```python
from build123d import *

# Parameters (mm, degrees)
F1_DEPTH      = 25.4
F2_T          = -2.54
F8_DEPTH      = 12.7
F8_DEPTH_BACK = 25.4


# Not quite as in the source:
# - the program builds the solid bodies; features that only make, move or delete a surface that nothing else refers to are left out


with BuildPart() as f1:
    # F0 (on Top) → F1 (new body)
    with BuildSketch(Plane.XY):
        Polygon((10.2551429075, 58.9377772835), (-40.5448570925, 58.9377772835), (-71.7704754875, 18.8678289949), (-41.2404706852, -21.7346192906), (9.5595293148, -21.7346192906), (40.7851477097, 18.335328998), align=None)
    extrude(amount=F1_DEPTH)

    # F2
    f2_openings = [f1.faces().sort_by_distance(p)[0] for p in [
        (-15.492664, 18.601579, 25.4),
    ]]
    offset(amount=F2_T, openings=f2_openings)

    # F7 (on Top) → F8 (join, two sides)
    with BuildSketch(Plane.XY) as f8_sk:
        Polygon((0, 0), (-50.8, 0), (-38.1, -21.9970452561), (-12.7, -21.9970452561), align=None)
    extrude(amount=F8_DEPTH)
    extrude(f8_sk.sketch, amount=-F8_DEPTH_BACK)


solid = f1.part
```
Build history of the part. All positions in model axes, mm. A direction names the side the tool comes from. Give positions to 0.01 mm unless a question says otherwise; leave off trailing zeros. Order: outer loops, then holes, each group sorted by start corner. A loop starts at its lowest first (then second) coordinate and runs counter-clockwise, first axis right, second up. Notation, with made-up numbers: M 30,89.25 L 61,89.25 A29 ccw 61,117.25 Z; hole C -20.5,41 d11. An arc over 180 degrees is marked long. Write item = value, one per line. Start each with the question number.
(1) Slice it at D-D on z = -14.5. Write the cut outline in (x, y).
(2) Probe L1, parallel to Z at x = -57.5, y = 33.5; L2, parallel to Z at x = 20, y = 23.5; L3, parallel to Y at x = -36, z = -14. List the from-to ranges inside material, lowest first. Write a range as [from, to].
(3) Pin check, flat tips, straight feed: pin 1 Ø1.5 at (y, z) = (30, 13.5) entering from -X; pin 2 Ø2 at (y, z) = (-11, -0.5) entering from -X; pin 3 Ø4 at (x, z) = (-39, -14.5) entering from +Y. Stop position of each tip, or through.
(4) Which spindle directions (+Z, -Z, +X, -X, +Y, -Y) get a long thin tool onto all of the face, cutting with end or side? Do faces 1 (the flat face through (-54.472, 0.089, 13.81)), 2 (the flat face through (-15, 58.938, 13)), 3 (the flat face through (-25, 0, -13)). Say none if no direction does.
(5) Slice it at A-A on z = 7. Write the cut outline in (x, y), plus the area to 3 significant figures.
(6) Slice it at B-B on x = -36. Write the cut outline in (y, z).
(7) Two-plate mould, pull along X, no slides. Class faces 4 (the flat face through (-16, 58, 25.4)), 5 (the flat face through (-55.94, 39.18, 12.52)), 6 (the flat face through (22.748, -0.679, 13.81)): released by +X, released by -X, zero draft, split by the parting line, or undercut.
(8) Slice it at C-C on y = 28.5. Write the cut outline in (x, z), plus the area to 3 significant figures.
Responses:
q1.outline = M -50.8,0 L -38.1,-22 L -12.7,-22 L 0,0 Z
q2.L1 = [0, 25.4]
q2.L2 = [0, 2.54]
q2.L3 = [-22, 0]
q3.pin_1 = -63.68
q3.pin_2 = -49.96
q3.pin_3 = 0
q4.face_1 = +Z
q4.face_2 = +Z, -Z, +X, -X, +Y
q4.face_3 = -Z, +X, -X, +Y
q5.outline = M -71.77,18.87 L -41.24,-21.73 L -38.25,-21.73 L -38.1,-22 L -12.7,-22 L -12.55,-21.73 L 9.56,-21.73 L 40.79,18.34 L 10.26,58.94 L -40.54,58.94 Z; hole M -68.57,18.84 L -39.97,-19.19 L -39.72,-19.19 L -50.8,0 L 0,0 L -11.08,-19.19 L 8.32,-19.19 L 37.59,18.36 L 8.99,56.4 L -39.3,56.4 Z
q5.area = 1,520 mm2
q6.outline = M -22,-25.4 L 0,-25.4 L 0,0 L 58.94,0 L 58.94,25.4 L 56.4,25.4 L 56.4,2.54 L 0,2.54 L 0,12.7 L -19.19,12.7 L -19.19,25.4 L -21.73,25.4 L -21.73,12.7 L -22,12.7 Z
q7.face_4 = zero draft
q7.face_5 = released by -X
q7.face_6 = undercut
q8.outline = M -64.26,0 L 33.14,0 L 33.14,25.4 L 29.96,25.4 L 29.96,2.54 L -61.04,2.54 L -61.04,25.4 L -64.26,25.4 Z
q8.area = 394 mm2
